Input: part model. Units: mm. Frame: model coordinates. Face numbers are marked on the shaded views. A direction names the side the tool comes from. Coordinates: 2 decimals unless noted, no trailing zeros. Write each loop counter-clockwise with the first axis right and the second up, starting at its lowest first coordinate (ties: lowest second). Pieces come first, ordered by that corner, then holes. Notation, with made-up numbers: M 42.5,-32.5 L 46.5,-32.5 A14 ccw 46.5,-7.5 Z; hole C -8,70 d4. An arc over 180 degrees is marked long. Use one line per item in the form item = value.
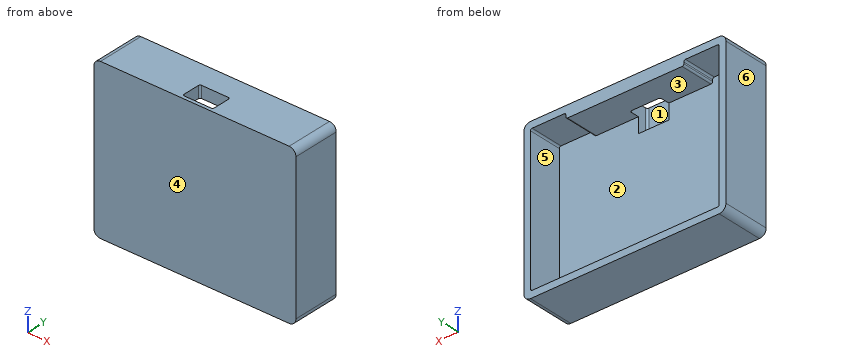
from build123d import *

# Parameters (mm, degrees)
SKETCH1_W               = 60
SKETCH1_H               = 47
BOSS_EXTRUDE1_DEPTH     = 4
SKETCH2_W               = 60
SKETCH2_H               = 47
SKETCH2_W_2             = 56
SKETCH2_H_2             = 43
BOSS_EXTRUDE2_DEPTH     = 10
SKETCH4_W               = 35
SKETCH4_H               = 12
BOSS_EXTRUDE3_DEPTH     = 1.5
CUT_EXTRUDE1_DEPTH      = 3
CUT_EXTRUDE1_DEPTH_BACK = 3
SKETCH5_W               = 9
SKETCH5_H               = 8
FILLET1_R               = 2
FILLET2_R               = 0.5
FILLET3_R               = 0.5


with BuildPart() as part:
    # Sketch1 → Boss-Extrude1 (new body)
    with BuildSketch(Plane(origin=(0, 0, 0), x_dir=(1, 0, 0), z_dir=(0, 1, 0))):
        Rectangle(SKETCH1_W, SKETCH1_H)
    extrude(amount=BOSS_EXTRUDE1_DEPTH)

    # Sketch2 → Boss-Extrude2 (add)
    with BuildSketch(Plane(origin=(0, 4, 0), x_dir=(1, 0, 0), z_dir=(0, 1, 0))):
        Rectangle(SKETCH2_W, SKETCH2_H)
        Rectangle(SKETCH2_W_2, SKETCH2_H_2, mode=Mode.SUBTRACT)
    extrude(amount=BOSS_EXTRUDE2_DEPTH)

    # Sketch4 → Boss-Extrude3 (add)
    with BuildSketch(Plane(origin=(0, 0, 21.5), x_dir=(-1, 0, 0), z_dir=(0, 0, -1))):
        with Locations((0, 8)):
            Rectangle(SKETCH4_W, SKETCH4_H)
    extrude(amount=BOSS_EXTRUDE3_DEPTH)

    # Sketch5 → Cut-Extrude1 (cut, two sides: drawn at the far end of the back side and taken through both)
    with BuildSketch(Plane(origin=(0, 4, 0), x_dir=(1, 0, 0), z_dir=(0, 1, 0)).offset(-CUT_EXTRUDE1_DEPTH_BACK)):
        with Locations((0, -19.5)):
            Rectangle(SKETCH5_W, SKETCH5_H)
    extrude(amount=CUT_EXTRUDE1_DEPTH + CUT_EXTRUDE1_DEPTH_BACK, mode=Mode.SUBTRACT)

    # Fillet1
    fillet1_edges = [part.edges().sort_by_distance(p)[0] for p in [
        (30, 7, 23.5),
        (-30, 7, 23.5),
        (-30, 7, -23.5),
        (30, 7, -23.5),
    ]]
    fillet(fillet1_edges, radius=FILLET1_R)

    # Fillet2
    fillet2_edges = [part.edges().sort_by_distance(p)[0] for p in [
        (28, 9, -21.5),
        (-28, 9, -21.5),
        (-28, 9, 21.5),
        (28, 9, 21.5),
        (-17.5, 9, 21.5),
        (17.5, 9, 21.5),
        (17.5, 9, 20),
        (-17.5, 9, 20),
    ]]
    fillet(fillet2_edges, radius=FILLET2_R)

    # Fillet3
    fillet3_edges = [part.edges().sort_by_distance(p)[0] for p in [
        (4.5, 1, 19.5),
        (-4.5, 1, 19.5),
        (4.5, 7, 21.75),
        (-4.5, 7, 21.75),
    ]]
    fillet(fillet3_edges, radius=FILLET3_R)


solid = part.part
(1) Pull-direction query (Y, two-part tool) for the marked faces 1, 2, 3 and 4; classes: pulls with the +Y half, pulls with the -Y half, needs draft (parallel to the pull), parting line crosses it, or undercut.
Computed:
face_1 = undercut
face_2 = pulls with the +Y half
face_3 = needs draft
face_4 = pulls with the -Y half
(2) Section query B-B on x = 22. Return the cut outline in (y, z), plus the area to 3 significant figures.
Computed:
outline = M 0,-23.5 L 14,-23.5 L 14,-21.5 L 4,-21.5 L 4,21.5 L 14,21.5 L 14,23.5 L 0,23.5 Z
area = 228 mm^2
(3) Section query A-A on y = 4.75. Return the cut outline in (x, z).
Computed:
outline = M -30,-21.5 A2 ccw -28,-23.5 L 28,-23.5 A2 ccw 30,-21.5 L 30,21.5 A2 ccw 28,23.5 L 4.5,23.5 L 4.5,20 L 17,20 A0.5 ccw 17.5,20.5 L 17.5,21 A0.5 cw 18,21.5 L 27.5,21.5 A0.5 cw 28,21 L 28,-21 A0.5 cw 27.5,-21.5 L -27.5,-21.5 A0.5 cw -28,-21 L -28,21 A0.5 cw -27.5,21.5 L -18,21.5 A0.5 cw -17.5,21 L -17.5,20.5 A0.5 ccw -17,20 L -4.5,20 L -4.5,23.5 L -28,23.5 A2 ccw -30,21.5 Z
(4) Section query C-C on z = -3. Return the cut outline in (x, y).
Computed:
outline = M -30,0 L 30,0 L 30,14 L 28,14 L 28,4 L -28,4 L -28,14 L -30,14 Z
(5) Line query: probe 1 along X at (y, z) = (12.5, 15.5); probe 2 along Z at (x, y) = (18, 6.5); probe 3 along X at (y, z) = (8.5, 21). Output: solid intervals per line, ascending.
Computed:
probe_1 = -30 to -28, 28 to 30
probe_2 = -23.5 to -21.5, 21.5 to 23.5
probe_3 = -30 to -28, -17.5 to 17.5, 28 to 30
(6) Section query D-D on y = 11.75. Return the cut outline in (x, z), plus the area to 3 significant figures.
Computed:
outline = M -30,-21.5 A2 ccw -28,-23.5 L 28,-23.5 A2 ccw 30,-21.5 L 30,21.5 A2 ccw 28,23.5 L -28,23.5 A2 ccw -30,21.5 Z; hole M -28,-21 A0.5 ccw -27.5,-21.5 L 27.5,-21.5 A0.5 ccw 28,-21 L 28,21 A0.5 ccw 27.5,21.5 L 18,21.5 A0.5 ccw 17.5,21 L 17.5,20.5 A0.5 cw 17,20 L -17,20 A0.5 cw -17.5,20.5 L -17.5,21 A0.5 ccw -18,21.5 L -27.5,21.5 A0.5 ccw -28,21 Z
area = 461 mm^2
(7) Set-up query: the marked faces 5 and 6. Return all of +Z, -Z, +X, -X, +Y, -Y with unobstructed straight access to the full face (end or side cutting, diameter ignored); none if empty.
Computed:
face_5 = +Y
face_6 = +Z, -Z, -X, +Y, -Y
